Could you check a few things on this model? Use its own coordinates, in mm. Round coordinates to 2 decimals unless told otherwise and drop trailing zeros. Write each loop counter-clockwise with the first axis right and the second up, starting at its lowest first coordinate (ties: lowest second). Pieces come first, ordered by that corner, then holes. Notation, with made-up numbers: (-3, 0) -> (36, 0) arc R28 cw to (36, 22) -> close; hole circle Ø3 at (4.25, 32). An arc over 180 degrees is marked (long way). Answer as CSV lines item,"result". Start each with the question number.
Q1. Will these pins go through, and if not, where does the flat tip stop? pin 1 Ø6 at (x, y) = (70.5, 929.63) entering from +Z; pin 2 Ø1.5 at (x, z) = (-33.5, 0.5) entering from +Y; pin 3 Ø16 at (x, y) = (-14.5, 757.63) entering from -Z.
Q2. Imagine slicing it at A-A on y = 826.5. Please give me the cut outline in (x, z), and give its area (3 significant figures).
Q3. If I drill on line 1 (Y direction, x = -110.5, z = 2.15); line 2 (X direction, y = 909, z = 1.1); line 3 (Y direction, x = -15, z = 2.75), over which ranges is the centre line in solid material (lowest first)? Write a range as [from, to].
Q4. Imagine slicing it at B-B on x = -15.5. Please give me the cut outline in (y, z), and give its area (3 significant figures).
Q5. Imagine slicing it at C-C on z = 0.5. Give the number of separate pieces and of enclosed holes in the cut face, and give its area (3 significant figures).
Q6. Imagine slicing it at D-D on x = 25. Please give me the cut outline in (y, z).
from build123d import *

# Parameters (mm, degrees)
CROQUIS1_R              = 2.5
CROQUIS1_R_2            = 10
SALIENTE_EXTRUIR1_DEPTH = 3


with BuildPart() as part:
    # Croquis1 → Saliente-Extruir1 (new body)
    with BuildSketch(Plane.XY):
        Polygon((-79.498385096, 944.128389678), (-79.498385096, 777.628389678), (50.501614904, 777.628389678), (50.501614904, 944.128389678), (90.501614904, 944.128389678), (90.501614904, 703.628389678), (-119.498385096, 703.628389678), (-119.498385096, 944.128389678), align=None)
        with Locations((70.501614904, 929.628389678)):
            Circle(CROQUIS1_R, mode=Mode.SUBTRACT)
        with Locations((81.501614904, 875.618389678)):
            Circle(CROQUIS1_R, mode=Mode.SUBTRACT)
        with Locations((81.501614904, 783.618389678)):
            Circle(CROQUIS1_R, mode=Mode.SUBTRACT)
        with Locations((-36.165051763, 762.628389678)):
            Circle(CROQUIS1_R, mode=Mode.SUBTRACT)
        with Locations((-110.498385096, 783.618389678)):
            Circle(CROQUIS1_R, mode=Mode.SUBTRACT)
        with Locations((-110.498385096, 875.618389678)):
            Circle(CROQUIS1_R, mode=Mode.SUBTRACT)
        with Locations((-99.498385096, 929.628389678)):
            Circle(CROQUIS1_R, mode=Mode.SUBTRACT)
        with Locations((7.168281571, 762.628389678)):
            Circle(CROQUIS1_R, mode=Mode.SUBTRACT)
        with Locations((-14.498385096, 757.628389678)):
            Circle(CROQUIS1_R_2, mode=Mode.SUBTRACT)
    extrude(amount=SALIENTE_EXTRUIR1_DEPTH)


solid = part.part
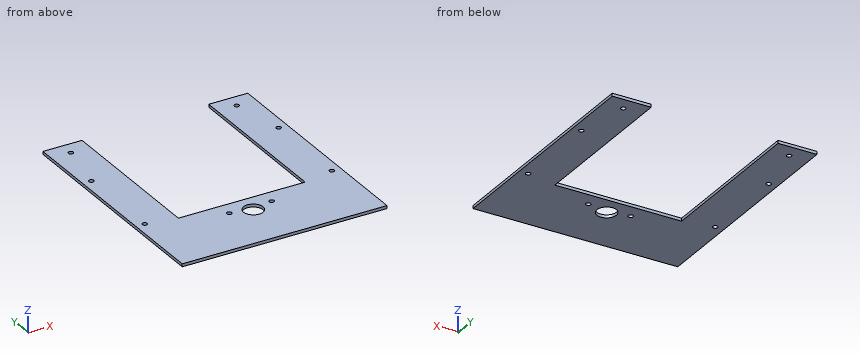
Checks:
1,pin 1,"z = 3"
1,pin 2,"y = 777.63"
1,pin 3,"through"
2,outline,"(-119.5, 0) -> (-79.5, 0) -> (-79.5, 3) -> (-119.5, 3) -> close; (50.5, 0) -> (90.5, 0) -> (90.5, 3) -> (50.5, 3) -> close"
2,area,"240 mm^2"
3,line 1,"[703.63, 781.12], [786.12, 873.12], [878.12, 944.13]"
3,line 2,"[-119.5, -79.5], [50.5, 90.5]"
3,line 3,"[703.63, 747.64], [767.62, 777.63]"
4,outline,"(703.63, 0) -> (747.68, 0) -> (747.68, 3) -> (703.63, 3) -> close; (767.58, 0) -> (777.63, 0) -> (777.63, 3) -> (767.58, 3) -> close"
4,area,"162 mm^2"
5,separate pieces,"1"
5,enclosed holes,"9"
5,area,"28,400 mm^2"
6,outline,"(703.63, 0) -> (777.63, 0) -> (777.63, 3) -> (703.63, 3) -> close"
